Model file for the job. Use its own axes, mm. Face numbers are marked on the shaded views. A direction names the side the tool comes from. Round coordinates to 2 decimals unless told otherwise and drop trailing zeros. Loops run counter-clockwise (first coordinate to the right, second up) from the corner with the lowest first, then second, coordinate; pieces in that order, holes last. Notation, with made-up numbers: (72, 40.25) - (103, 40.25) arc R5 cw to (103, 45.25) - close; hole circle Ø4 at (26, 46). An arc over 180 degrees is marked (long way). Use one line per item in the form item = value.
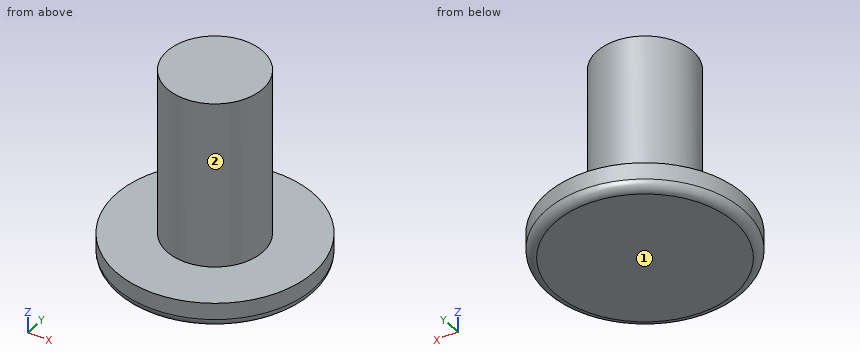
from build123d import *

# Parameters (mm, degrees)
SKETCH1_R           = 5.56
BOSS_EXTRUDE1_DEPTH = 1.44
SKETCH2_R           = 2.69
BOSS_EXTRUDE2_DEPTH = 9.43
FILLET1_R           = 0.5


with BuildPart() as part:
    # Sketch1 → Boss-Extrude1 (new body)
    with BuildSketch(Plane.XY):
        Circle(SKETCH1_R)
    extrude(amount=BOSS_EXTRUDE1_DEPTH)

    # Sketch2 → Boss-Extrude2 (add)
    with BuildSketch(Plane.XY.offset(1.44)):
        Circle(SKETCH2_R)
    extrude(amount=BOSS_EXTRUDE2_DEPTH)

    # Fillet1
    fillet1_edges = [part.edges().sort_by_distance(p)[0] for p in [
        (-5.56, 0, 0),
    ]]
    fillet(fillet1_edges, radius=FILLET1_R)


solid = part.part
1. Wall check: probe 1 along Z at (x, y) = (-3.75, 2.5); probe 2 along Y at (x, z) = (4.5, 0.5); probe 3 along X at (y, z) = (-4, 0.75). Give the ranges that are in metal, low to high.
Geometry check:
probe_1 = 0 to 1.44
probe_2 = -3.27 to 3.27
probe_3 = -3.86 to 3.86
2. Flat gauge pins, fed straight in: pin 1 (1 mm diameter, centred on x = -0.5, z = 3, fed in from +Y); pin 2 (6 mm diameter, centred on x = 1, z = 9.5, fed in from -Y). Where does each tip first touch, or does it go through?
Geometry check:
pin_1 = 2.69
pin_2 = -2.69
3. Tool access for the marked faces 1 and 2: list every direction of +Z, -Z, +X, -X, +Y, -Y with a clear straight run to the whole face (end or side of a thin tool).
Geometry check:
face_1 = -Z, +X, -X, +Y, -Y
face_2 = +Z
4. Cut at A-A, the plane x = 0. Give the cut face in (y, z).
Geometry check:
outline = (-5.56, 0.5) arc R0.5 ccw to (-5.06, 0) - (5.06, 0) arc R0.5 ccw to (5.56, 0.5) - (5.56, 1.44) - (2.69, 1.44) - (2.69, 10.87) - (-2.69, 10.87) - (-2.69, 1.44) - (-5.56, 1.44) - close
5. Cut at C-C, the plane z = 4. Give the cut face in (x, y), plus the area to 3 significant figures.
Geometry check:
outline = circle Ø5.38 at (0, 0)
area = 22.7 mm^2
